Geometry: final body of the model. Coordinates: model frame, mm. Face numbers are marked on the shaded views. A direction names the side the tool comes from. Give positions to 0.01 mm unless a question says otherwise; leave off trailing zeros. Loops run counter-clockwise (first coordinate to the right, second up) from the corner with the lowest first, then second, coordinate; pieces in that order, holes last. Notation, with made-up numbers: M 10,70 L 66,70 A17 ccw 66,87 Z; hole C 24,48 d3. An arc over 180 degrees is marked long. Put each result on its own line as item: value.
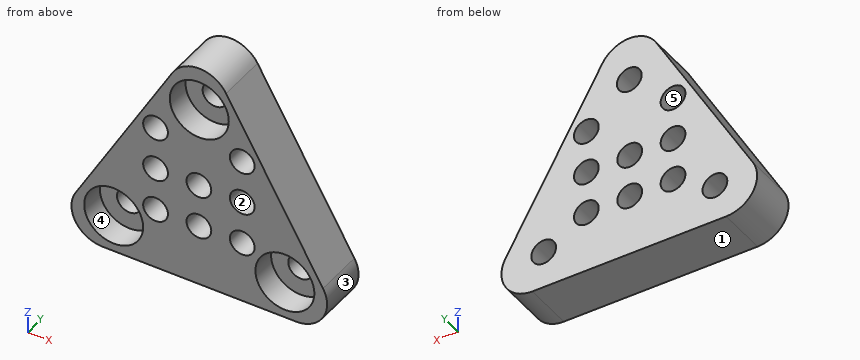
```python
from build123d import *

# Parameters (mm, degrees)
SKETCH1_R      = 1
EXTRUDE1_DEPTH = 4
SKETCH1_3_R    = 2.38125
EXTRUDE4_DEPTH = 2


with BuildPart() as part:
    # Sketch1 → Extrude1 (new body)
    with BuildSketch(Plane(origin=(0, 0, 0), x_dir=(1, 0, 0), z_dir=(0, 1, 0))):
        with BuildLine():
            Line((-5.186041147, 3.316192399), (2.637731834, -10.234979911))
            ThreePointArc((2.637731834, -10.234979911), (4.802795343, -11.484979911), (6.967858853, -10.234979911))
            Line((6.967858853, -10.234979911), (14.791631834, 3.316192399))
            ThreePointArc((14.791631834, 3.316192399), (14.791631834, 5.816192399), (12.626568324, 7.066192399))
            Line((12.626568324, 7.066192399), (-3.020977638, 7.066192399))
            ThreePointArc((-3.020977638, 7.066192399), (-5.186041147, 5.816192399), (-5.186041147, 3.316192399))
        make_face()
        with Locations((-2.110635714, 4.040606244)):
            Circle(SKETCH1_R, mode=Mode.SUBTRACT)
        with Locations((11.7162264, 4.040606244)):
            Circle(SKETCH1_R, mode=Mode.SUBTRACT)
        with Locations((4.802795343, -7.933807601)):
            Circle(SKETCH1_R, mode=Mode.SUBTRACT)
        with Locations((1.270334632, 2.088602105)):
            Circle(SKETCH1_R, mode=Mode.SUBTRACT)
        with Locations((4.770334632, 2.088602105)):
            Circle(SKETCH1_R, mode=Mode.SUBTRACT)
        with Locations((8.270334632, 2.088602105)):
            Circle(SKETCH1_R, mode=Mode.SUBTRACT)
        with Locations((1.270334632, -1.411397895)):
            Circle(SKETCH1_R, mode=Mode.SUBTRACT)
        with Locations((4.770334632, -1.411397895)):
            Circle(SKETCH1_R, mode=Mode.SUBTRACT)
        with Locations((8.270334632, -1.411397895)):
            Circle(SKETCH1_R, mode=Mode.SUBTRACT)
        with Locations((1.270334632, -4.911397895)):
            Circle(SKETCH1_R, mode=Mode.SUBTRACT)
        with Locations((8.270334632, -4.911397895)):
            Circle(SKETCH1_R, mode=Mode.SUBTRACT)
    extrude(amount=EXTRUDE1_DEPTH)

    # Sketch1<3> → Extrude4 (cut)
    with BuildSketch(Plane(origin=(0, 0, 0), x_dir=(1, 0, 0), z_dir=(0, 1, 0))):
        with Locations((-2.110635714, 4.040606244)):
            Circle(SKETCH1_3_R)
        with Locations((4.802795343, -7.933807601)):
            Circle(SKETCH1_3_R)
        with Locations((11.7162264, 4.040606244)):
            Circle(SKETCH1_3_R)
    extrude(amount=EXTRUDE4_DEPTH, mode=Mode.SUBTRACT)


solid = part.part
```
Item 1: Mould query, pull axis Z, two halves, no side actions, for the marked faces 1, 2 and 3. Classes: pulls with the +Z half, pulls with the -Z half, needs draft (parallel to the pull), parting line crosses it, or undercut.
Output values:
face 1: pulls with the -Z half
face 2: undercut
face 3: parting line crosses it
Item 2: Section D-D on x = 13.5. Output: boundary loops of the cut face in (y, z), then the cut area to 3 significant figures.
Output values:
outline: M 0,-6.91 L 4,-6.91 L 4,-1.08 L 0,-1.08 L 0,-2.46 L 2,-2.46 L 2,-5.62 L 0,-5.62 Z
area: 17.0 mm²
Item 3: Pin query (flat end, axial travel): pin 1 Ø2.5 at (x, z) = (4.77, -2.09) entering from +Y; pin 2 Ø1.5 at (y, z) = (2.5, -0.5) entering from +X; pin 3 Ø2 at (x, y) = (7.5, 1) entering from +Z; pin 4 Ø4 at (x, z) = (11.72, -4.04) entering from -Y. Return the tip coordinate at first contact, or that it passes through.
Output values:
pin 1: y = 4
pin 2: x = 13.6
pin 3: z = 10.82
pin 4: y = 2
Item 4: Section B-B on z = 4.5. Output: boundary loops of the cut face in (x, y).
Output values:
outline: M -0.67,0 L 0.36,0 L 0.36,4 L -0.67,4 Z; M 2.18,0 L 7.36,0 L 7.36,4 L 2.18,4 Z; M 9.18,0 L 10.28,0 L 10.28,4 L 9.18,4 Z
Item 5: Section A-A on x = 1. Output: boundary loops of the cut face in (y, z).
Output values:
outline: M 0,-7.07 L 4,-7.07 L 4,-3.05 L 0,-3.05 Z; M 0,-1.13 L 4,-1.13 L 4,0.45 L 0,0.45 Z; M 0,2.37 L 4,2.37 L 4,3.95 L 0,3.95 Z; M 0,5.87 L 4,5.87 L 4,7.4 L 0,7.4 Z
Item 6: Set-up query: the marked faces 4 and 5. Return all of +Z, -Z, +X, -X, +Y, -Y with unobstructed straight access to the full face (end or side cutting, diameter ignored); none if empty.
Output values:
face 4: -Y
face 5: +Y, -Y
Item 7: Line query: probe 1 along X at (y, z) = (0.45, 4.5); probe 2 along Z at (x, y) = (1.75, 1.3); probe 3 along Z at (x, y) = (7.75, 3.4). Output: solid intervals per line, ascending. Write a range as [from, to].
Output values:
probe 1: [-0.67, 0.36], [2.18, 7.36], [9.18, 10.28]
probe 2: [-7.07, -2.97], [-1.21, 0.53], [2.29, 4.03], [5.79, 8.7]
probe 3: [-7.07, -2.94], [-1.23, 0.56], [2.27, 4.06], [5.77, 8.88]
Item 8: Section C-C on y = 0.65. Count the separate pieces of the cut face and the enclosed holes in it, then the cut area to 3 significant figures.
Output values:
separate pieces: 1
enclosed holes: 11
area: 164 mm²
